Could you check a few things on this model? Use its own coordinates, in mm. A direction names the side the tool comes from. Coordinates: 2 decimals unless noted, no trailing zeros. Order: outer loops, then holes, each group sorted by start corner. A loop starts at its lowest first (then second) coordinate and runs counter-clockwise, first axis right, second up. Notation, with made-up numbers: (2.5, 43) -> (26.5, 43) arc R17 ccw to (26.5, 56) -> close; hole circle Ø10 at (-4.5, 57). An arc over 180 degrees is marked (long way). Use a Markdown table: item, result. Add a question column.
1) If we section it at D-D (x = 3): Write out the boundary of the cut face in (y, z).
2) If we section it at C-C (z = 6.25): Write out the boundary of the cut face in (x, y), plus the area to 3 significant figures.
3) Which directions (+Z, -Z, +X, -X, +Y, -Y) give clear straight access to the entire face, cutting with the end or side of a thin tool? Please do faces 1 (the flat face through (3, -1, 0)), 2 (the flat face through (3, -3, 9)).
4) If I drill on L1, parallel to Y at x = 0, z = 4; L2, parallel to Y at x = 0, z = 9.75; L3, parallel to X at y = -2, z = 8.75, over which ranges is the centre line in solid material (lowest first)? Write a range as [from, to].
5) If we section it at A-A (x = 0): Write out the boundary of the cut face in (y, z).
6) Will these pins go through, and if not, where does the flat tip stop? pin 1 Ø1 at (y, z) = (1, 3) entering from +X; pin 2 Ø6 at (x, z) = (1, 2) entering from -Y; pin 3 Ø2 at (y, z) = (-2.5, 3.5) entering from +X.
7) Thinking about a two-plate mould opening in Y: for faces 3 (the flat face through (2, -2, 14)), 4 (the cylindrical face through (2.45, -1.01, 6.9)), 5 (the cylindrical face through (-2.87, 2.64, 4.44)), which applies, +Y half, -Y half, draft (parallel to the pull), parting line (faces both ways), or undercut?
```python
from build123d import *

# Parameters (mm, degrees)
SCHIZZO1_R                   = 3.9
SCHIZZO1_R_2                 = 2.65
ESTRUSIONE_ESTRUSIONE1_DEPTH = 9
SCHIZZO2_R                   = 5
SCHIZZO2_R_2                 = 3.9
ESTRUSIONE_ESTRUSIONE3_DEPTH = 5
SCHIZZO3_R                   = 3.9
SCHIZZO3_R_2                 = 2.65
ESTRUSIONE_ESTRUSIONE4_DEPTH = 5


with BuildPart() as part:
    # Schizzo1 → Estrusione-Estrusione1 (new body)
    with BuildSketch(Plane.XY):
        Circle(SCHIZZO1_R)
        Circle(SCHIZZO1_R_2, mode=Mode.SUBTRACT)
    extrude(amount=ESTRUSIONE_ESTRUSIONE1_DEPTH)



with BuildPart() as body_2:
    # Schizzo2 → Estrusione-Estrusione3 (new body)
    with BuildSketch(Plane.XY.offset(9)):
        Circle(SCHIZZO2_R)
        Circle(SCHIZZO2_R_2, mode=Mode.SUBTRACT)
    extrude(amount=ESTRUSIONE_ESTRUSIONE3_DEPTH)


with BuildPart() as part_1:
    add(part.part)

    add(body_2.part)  # Estrusione-Estrusione4 merges body 2
    # Schizzo3 → Estrusione-Estrusione4 (add)
    with BuildSketch(Plane.XY.offset(9)):
        Circle(SCHIZZO3_R)
        Circle(SCHIZZO3_R_2, mode=Mode.SUBTRACT)
    extrude(amount=ESTRUSIONE_ESTRUSIONE4_DEPTH)


solid = part_1.part
```
Answer sheet:
| question | item | result |
|---|---|---|
| 1 | outline | (-4, 9) -> (-2.49, 9) -> (-2.49, 0) -> (2.49, 0) -> (2.49, 9) -> (4, 9) -> (4, 14) -> (-4, 14) -> close |
| 2 | outline | circle Ø7.8 at (0, 0); hole circle Ø5.3 at (0, 0) |
| 2 | area | 25.7 mm2 |
| 3 | face 1 | -Z, +X, -X, +Y, -Y |
| 3 | face 2 | -Z |
| 4 | L1 | [-3.9, -2.65], [2.65, 3.9] |
| 4 | L2 | [-5, -2.65], [2.65, 5] |
| 4 | L3 | [-3.35, -1.74], [1.74, 3.35] |
| 5 | outline | (-5, 9) -> (-3.9, 9) -> (-3.9, 0) -> (-2.65, 0) -> (-2.65, 14) -> (-5, 14) -> close; (2.65, 0) -> (3.9, 0) -> (3.9, 9) -> (5, 9) -> (5, 14) -> (2.65, 14) -> close |
| 6 | pin 1 | x = 3.87 |
| 6 | pin 2 | y = -3.9 |
| 6 | pin 3 | x = 3.6 |
| 7 | face 3 | draft |
| 7 | face 4 | undercut |
| 7 | face 5 | parting line |
